from build123d import *

# Parameters (mm, degrees)
SKETCH1_W           = 84
SKETCH1_H           = 300
SKETCH1_W_2         = 54
SKETCH1_H_2         = 80
BOSS_EXTRUDE1_DEPTH = 6
SKETCH2_R           = 1
CUT_EXTRUDE1_DEPTH  = 10
SKETCH4_R           = 1
CUT_EXTRUDE3_DEPTH  = 10
SKETCH5_R           = 1
CUT_EXTRUDE4_DEPTH  = 10


with BuildPart() as part:
    # Sketch1 → Boss-Extrude1 (new body)
    with BuildSketch(Plane.XY):
        Rectangle(SKETCH1_W, SKETCH1_H)
        with Locations((0, 95)):
            Rectangle(SKETCH1_W_2, SKETCH1_H_2, mode=Mode.SUBTRACT)
        with Locations((0, -95)):
            Rectangle(SKETCH1_W_2, SKETCH1_H_2, mode=Mode.SUBTRACT)
        Rectangle(SKETCH1_W_2, SKETCH1_H_2, mode=Mode.SUBTRACT)
    extrude(amount=BOSS_EXTRUDE1_DEPTH)

    # Sketch2 → Cut-Extrude1 (cut)
    with BuildSketch(Plane(origin=(42, 0, 0), x_dir=(0, 0, -1), z_dir=(1, 0, 0))):
        with Locations((-3, 146)):
            Circle(SKETCH2_R)
        with Locations((-3, 0)):
            Circle(SKETCH2_R)
        with Locations((-3, -146)):
            Circle(SKETCH2_R)
        with Locations((-3, -292)):
            Circle(SKETCH2_R)
    cut_extrude1 = extrude(amount=-CUT_EXTRUDE1_DEPTH, mode=Mode.SUBTRACT)

    # Mirror1: Cut-Extrude1 across plane
    add(cut_extrude1.mirror(Plane(origin=(0, 0, 0), x_dir=(0, 0, 1), z_dir=(1, 0, 0))), mode=Mode.SUBTRACT)

    # Sketch4 → Cut-Extrude3 (cut)
    with BuildSketch(Plane.XY.offset(6)):
        with Locations((-37, 70)):
            Circle(SKETCH4_R)
        with Locations((-37, 20)):
            Circle(SKETCH4_R)
        with Locations((-37, -50)):
            Circle(SKETCH4_R)
        with Locations((-37, -110)):
            Circle(SKETCH4_R)
        with Locations(Location((37, -110, 0), (0, 0, 180))):
            Circle(SKETCH4_R)
        with Locations(Location((37, -50, 0), (0, 0, 180))):
            Circle(SKETCH4_R)
        with Locations(Location((37, 20, 0), (0, 0, 180))):
            Circle(SKETCH4_R)
        with Locations(Location((37, 70, 0), (0, 0, 180))):
            Circle(SKETCH4_R)
    extrude(amount=-CUT_EXTRUDE3_DEPTH, mode=Mode.SUBTRACT)

    # Sketch5 → Cut-Extrude4 (cut)
    with BuildSketch(Plane.XY.offset(6)):
        with Locations((-36.5, -140.5)):
            Circle(SKETCH5_R)
        with Locations((36.5, -140.5)):
            Circle(SKETCH5_R)
        with Locations((-36.5, 139.5)):
            Circle(SKETCH5_R)
        with Locations((36.5, 139.5)):
            Circle(SKETCH5_R)
    extrude(amount=-CUT_EXTRUDE4_DEPTH, mode=Mode.SUBTRACT)


solid = part.part
Can you work these out from the model? Positions are in its coordinate system, mm. A direction names the side the tool comes from. Round coordinates to 2 decimals unless told otherwise and drop trailing zeros. Write each loop counter-clockwise with the first axis right and the second up, starting at its lowest first coordinate (ties: lowest second). Pieces come first, ordered by that corner, then holes. Notation, with made-up numbers: (-3.75, 75) -> (47.25, 75) arc R18 cw to (47.25, 95) -> close; hole circle Ø7 at (40.5, -34). An arc over 180 degrees is marked (long way). One line per question, with ' | ' between items. Start each with the question number.
1) I'm going to push a flat-ended pin straight in: P1, Ø1.8, axis at y = 0, z = 3, coming from the +X side. Where does the tip first touch, or does it pass through?
2) If we mould it in two halves opening along Y, with no side actions, what happens to faces 1 (the flat face through (0, 135, 3)), 2 (the flat face through (-1, -150, 3)), 3 (the flat face through (0, -55, 3)), 4 (the flat face through (42, -2, 3))? For each: released by +Y, released by -Y, zero draft, split by the parting line, or undercut.
3) I need wall thicknesses on line 1 (Y direction, x = -7, z = 5.5); line 2 (Y direction, x = 40.25, z = 3); line 3 (X direction, y = 8.5, z = 2). Which ranges of each line are inside material? Lowest first, please. Write a range as [from, to].
4) Suppose I cut it at B-B on y = -21.5. Write out the boundary of the cut face in (x, z), then the cut area to 3 significant figures.
5) On a 3-axis mill with a long thin cutter (end or side, diameter ignored), from which of +Z, -Z, +X, -X, +Y, -Y can I reach the whole of each face in a straight line? I mean faces 5 (the flat face through (27, -96, 3)), 6 (the flat face through (-42, -2, 3)). Say none if no direction works.
6) Suppose I cut it at A-A on x = -5.5. Write out the boundary of the cut face in (y, z).
Return value:
1) P1: stops at x = 32
2) face 1: undercut | face 2: released by -Y | face 3: undercut | face 4: zero draft
3) line 1: y = [-150, -135], [-55, -40], [40, 55], [135, 150] | line 2: y = [-150, -147], [-145, -1], [1, 145], [147, 150] | line 3: x = [-42, -27], [27, 42]
4) outline: (-42, 0) -> (-27, 0) -> (-27, 6) -> (-42, 6) -> close; (27, 0) -> (42, 0) -> (42, 6) -> (27, 6) -> close | area: 180 mm2
5) face 5: +Z, -Z | face 6: +Z, -Z, -X, +Y, -Y
6) outline: (-150, 0) -> (-135, 0) -> (-135, 6) -> (-150, 6) -> close; (-55, 0) -> (-40, 0) -> (-40, 6) -> (-55, 6) -> close; (40, 0) -> (55, 0) -> (55, 6) -> (40, 6) -> close; (135, 0) -> (150, 0) -> (150, 6) -> (135, 6) -> close
